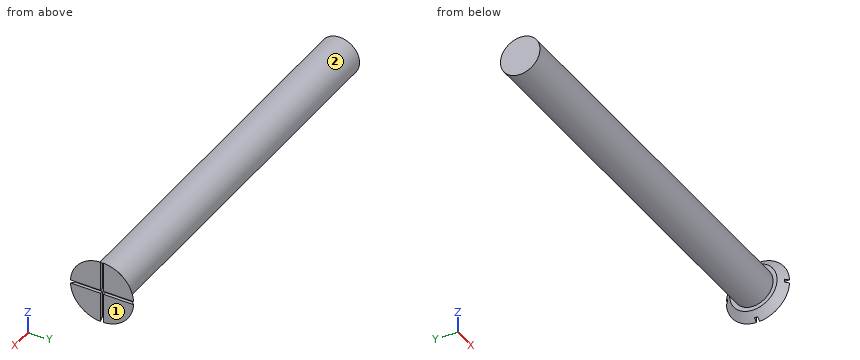
Autodesk Inventor part; units mm, degrees
ref_plane "YZ Plane" through (0, 0, 0) normal (1, 0, 0) x (0, 1, 0)
ref_plane "XZ Plane" through (0, 0, 0) normal (0, 1, 0) x (-1, 0, 0)
ref_plane "XY Plane" through (0, 0, 0) normal (0, 0, 1) x (1, 0, 0)
sketch "Sketch1" plane through (0, 0, 0) normal (1, 0, 0) x (0, 1, 0)
  circle A0 centre (0, 0) radius 3.175
  dimension "d0" = 6.35
extrude "Extrusion1" add sketch "Sketch1" against normal blind 63.5
sketch "Sketch2" plane through (0, 0, 0) normal (1, 0, 0) x (0, 0, -1)
  circle A0 centre (0, 0) radius 3.175
  circle A1 centre (0, 0) radius 5.08
  dimension "d3" = 10.16
extrude "Extrusion2" add sketch "Sketch2" along normal blind 1.27 contours A0 | A1
chamfer "Chamfer1" distance 1.27 angle 45 1 edges at (0, 0, 5.08)
sketch "Sketch3" plane through (1.27, 0, 0) normal (1, 0, 0) x (0, 0, -1)
  line L0 (-0.254, -5.08) -> (0.254, -5.08)
  line L1 (0.254, -5.08) -> (0.254, 5.08)
  line L2 (0.254, 5.08) -> (-0.254, 5.08)
  line L3 (-0.254, 5.08) -> (-0.254, -5.08)
  line L4 (-0.254, -5.08) -> (0.254, 5.08) construction
  line L5 (0.254, -5.08) -> (-0.254, 5.08) construction
  line L6 (-5.08, -0.254) -> (5.08, -0.254)
  line L7 (5.08, -0.254) -> (5.08, 0.254)
  line L8 (5.08, 0.254) -> (-5.08, 0.254)
  line L9 (-5.08, 0.254) -> (-5.08, -0.254)
  line L10 (-5.08, -0.254) -> (5.08, 0.254) construction
  line L11 (5.08, -0.254) -> (-5.08, 0.254) construction
  point P0 (0, 0)
  dimension "d9" = 0.508
  dimension "d10" = 10.16
  dimension "d11" = 10.16
  dimension "d12" = 0.508
extrude "Extrusion3" cut sketch "Sketch3" against normal blind 0.508
thread "Thread1"
properties part number "screws (for assembly)"
Work out the finished part from the listing and answer in its coordinate system (mm). Face numbers are marked on the shaded views. A direction names the side the tool comes from. Round coordinates to 2 decimals unless told otherwise and drop trailing zeros. Write each loop counter-clockwise with the first axis right and the second up, starting at its lowest first coordinate (ties: lowest second). Pieces come first, ordered by that corner, then holes. Notation, with made-up numbers: (-14, 14) - (37, 14) arc R21 cw to (37, 35) - close; hole circle Ø7 at (44.5, 84). An arc over 180 degrees is marked (long way). Answer in a Markdown table with one row per item. Add a question column.
1. Given pin 1 (3 mm diameter, centred on x = -34.5, z = 1.5, fed in from +Y) (3 decimals); pin 2 (2 mm diameter, centred on x = -43, y = 1, fed in from -Z) (3 decimals); pin 3 (3 mm diameter, centred on x = -40.5, y = -3.5, fed in from +Z), each flat-ended and moving along its own axis, determine where each tip first touches the part or whether it passes through.
2. Find the intervals of material crossed by line 1 along X through (y, z) = (0, -1.75); line 2 along Z through (x, y) = (-52, 1.5); line 3 along Z through (x, y) = (-13.5, -2), in increasing order. Write a range as from..to.
3. A cutting plane is placed at A-A, the plane x = -29.5. Determine the outline of the cut face in (y, z) (3 decimals), and give its area (3 significant figures).
4. For the marked faces 1 and 2, determine the directions among +Z, -Z, +X, -X, +Y, -Y from which every point of the face is accessible in a straight line to the end or side of a thin tool.
Worked out:
| question | item | result |
|---|---|---|
| 1 | pin 1 | y = 3.175 |
| 1 | pin 2 | z = -3.175 |
| 1 | pin 3 | z = 2.47 |
| 2 | line 1 | -63.5..0.76 |
| 2 | line 2 | -2.8..2.8 |
| 2 | line 3 | -2.47..2.47 |
| 3 | outline | circle Ø6.35 at (0, 0) |
| 3 | area | 31.7 mm^2 |
| 4 | face 1 | +Z, -Z, +X, +Y, -Y |
| 4 | face 2 | -X |
